Build history of the part. All positions in model axes, mm. A direction names the side the tool comes from. Round coordinates to 2 decimals unless told otherwise and drop trailing zeros. Write each loop counter-clockwise with the first axis right and the second up, starting at its lowest first coordinate (ties: lowest second). Pieces come first, ordered by that corner, then holes. Notation, with made-up numbers: M -2.75,28 L 18.25,28 A27 cw 18.25,48 Z; hole C -0.75,-19.75 d11. An arc over 180 degrees is marked long. Write item = value, one per line.
Autodesk Inventor part; units mm, degrees
ref_plane "Work Plane1" through (0, 54.4, 0) normal (0, 1, 0) x (1, 0, 0)
ref_plane "YZ Plane" through (0, 0, 0) normal (1, 0, 0) x (0, 1, 0)
ref_plane "XZ Plane" through (0, 0, 0) normal (0, 1, 0) x (-1, 0, 0)
sketch "Sketch1" plane through (0, 0, 0) normal (0, 1, 0) x (-1, 0, 0)
  circle A0 centre (0, 0) radius 4
  dimension "d0" = 8
extrude "Extrusion1" add sketch "Sketch1" along normal blind 50
chamfer "Chamfer1" distance 1 angle 45 1 edges at (4, 0, 0)
ref_plane "Work Plane1" through (0, 54.4, 0) normal (0, 1, 0) x (1, 0, 0)
thread "Thread1"
sketch "Sketch5" plane through (0, 50, 0) normal (0, 1, 0) x (1, 0, 0)
  circle A0 centre (0, 0) radius 7
  dimension "d17" = 14
sketch "Sketch6" plane through (0, 54.4, 0) normal (0, 1, 0) x (1, 0, 0)
  circle A0 centre (0, 0) radius 4
  dimension "d18" = 8
loft "Loft2" add profiles "Sketch5", "Sketch6"
fillet "Fillet1" radius 2 1 edges at (-4, 54.4, 0)
sketch "Sketch7" plane through (0, 54.4, 0) normal (0, 1, 0) x (1, 0, 0)
  line L0 (2.8868, 0) -> (1.4434, -2.5)
  line L1 (1.4434, -2.5) -> (-1.4434, -2.5)
  line L2 (-1.4434, -2.5) -> (-2.8868, 0)
  line L3 (-2.8868, 0) -> (-1.4434, 2.5)
  line L4 (-1.4434, 2.5) -> (1.4434, 2.5)
  line L5 (1.4434, 2.5) -> (2.8868, 0)
  point P0 (0, 0)
  point P1 (0, 0)
  dimension "d24" = 5
extrude "Extrusion3" cut sketch "Sketch7" against normal blind 5
properties part number "M8x50"
1. Band-saw the part on B-B (y = 17). List the corners of the cut face in (x, z), plus the area to 3 significant figures.
Responses:
outline = C 0,0 d8
area = 50.3 mm²
2. Flat gauge pins, fed straight in: pin 1 (8 mm diameter, centred on y = 19, z = 3.5, fed in from -X); pin 2 (8 mm diameter, centred on x = 5, y = 28, fed in from -Z); pin 3 (4 mm diameter, centred on x = 0, y = 40.5, fed in from -Z). Where does each tip first touch, or does it go through?
Responses:
pin_1 = -4
pin_2 = -3.87
pin_3 = -4
3. Probe probe 1 along Y at (x, z) = (0.75, 2.25); probe 2 along X at (y, z) = (13, 0.25); probe 3 along X at (y, z) = (15, 3.5). List the from-to ranges inside material, lowest first.
Responses:
probe_1 = 0 to 49.4
probe_2 = -3.99 to 3.99
probe_3 = -1.94 to 1.94
4. Tool access for faces 1 (the face through (0, 0, 0)), 2 (the face through (3, 50, 3)), 3 (the face through (2.175, 51.935, 1.233)): list every direction of +Z, -Z, +X, -X, +Y, -Y with a clear straight run to the whole face (end or side of a thin tool).
Responses:
face_1 = +Z, -Z, +X, -X, -Y
face_2 = -Y
face_3 = +Y
5. Band-saw the part on A-A (x = 0). List the corners of the cut face in (y, z), plus the area to 3 significant figures.
Responses:
outline = M 0,-3 L 1,-4 L 50,-4 L 50,-7 L 53.53,-4.6 A2 ccw 54.4,-2.94 L 54.4,-2.5 L 49.4,-2.5 L 49.4,2.5 L 54.4,2.5 L 54.4,2.94 A2 ccw 53.53,4.6 L 50,7 L 50,4 L 1,4 L 0,3 Z
area = 422 mm²
